Print and shaded views of the part. All mm, measured from the part's lowest x, y and z. A direction names the side the tool comes from. Round coordinates to 2 decimals unless told otherwise and drop trailing zeros. Write each loop counter-clockwise with the first axis right and the second up, starting at its lowest first coordinate (ties: lowest second). Pieces come first, ordered by that corner, then holes. Notation, with made-up numbers: M -35,81.5 L 7,81.5 A30 cw 7,114.5 Z; hole C -0.5,-26 d9. An arc over 180 degrees is marked long. Write item = value, one per line. Start each with the question number.
Q1. Probe L1, parallel to X at y = 15.25, z = 30.5; L2, parallel to Z at x = 44.5, y = 18.75; L3, parallel to Z at x = 54, y = 18.25. List the from-to ranges inside material, lowest first.
Q2. Band-saw the part on B-B on z = 36.5. Write the cut outline in (x, y), plus the area to 3 significant figures.
Q3. Pull direction Z, two halves, no side cores. Call the marked faces 1, 2, 3 and 4: released by +Z, released by -Z, zero draft, split by the parting line, or undercut.
Q4. Band-saw the part on C-C on y = 8.75. Write the cut outline in (x, z).
Q5. Band-saw the part on D-D on z = 10. Write the cut outline in (x, y), plus the area to 3 significant figures.
Q6. Drop flat-ended pins along their axis: P1, Ø2, axis at x = 13, y = 5, coming from the +Z side; P2, Ø4, axis at x = 38.5, y = 22.5, coming from the -Z side; P3, Ø6.5, axis at y = 13.5, z = 21, coming from the +X side. Give the stop position or say it passes through.
Q7. Tool access for the marked faces 5, 6, 7 and 8: list every direction of +Z, -Z, +X, -X, +Y, -Y with a clear straight run to the whole face (end or side of a thin tool).
Q8. Band-saw the part on A-A on x = 57.5. Write the cut outline in (y, z).
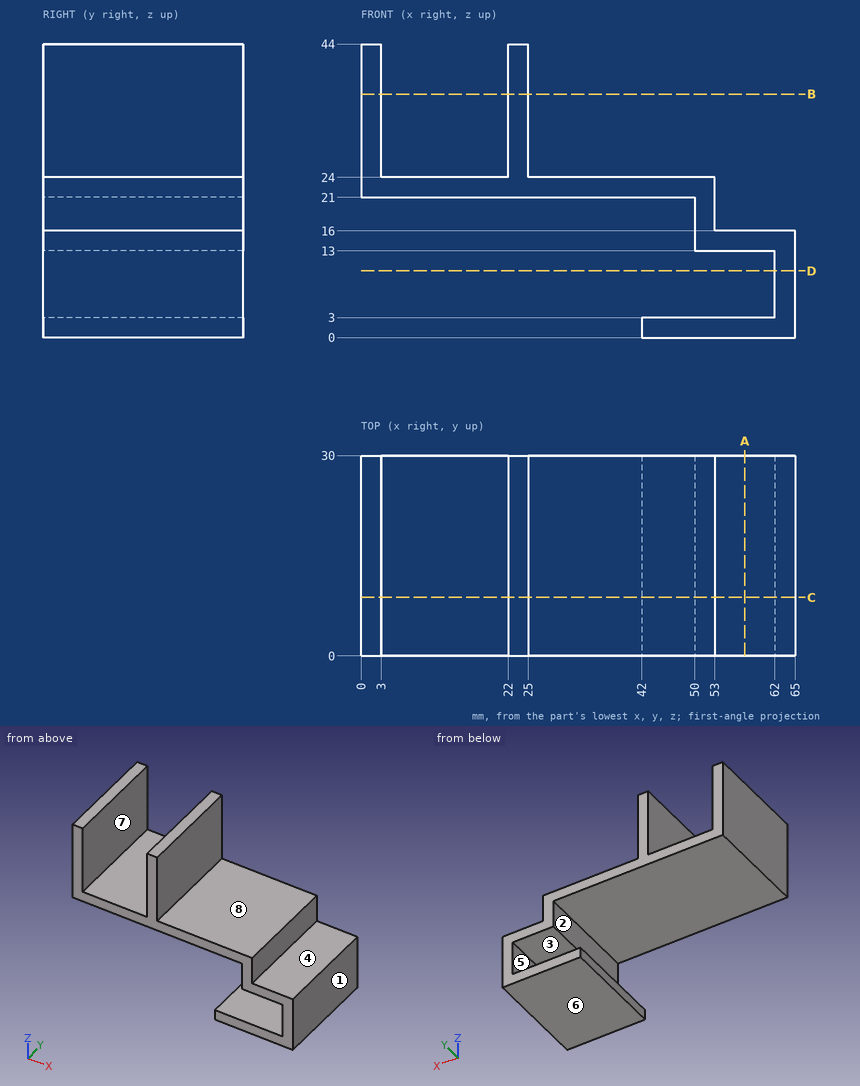
Conclusion:
q1.L1 = 0 to 3, 22 to 25
q1.L2 = 0 to 3, 21 to 24
q1.L3 = 0 to 3, 13 to 16
q2.outline = M 0,0 L 3,0 L 3,30 L 0,30 Z; M 22,0 L 25,0 L 25,30 L 22,30 Z
q2.area = 180 mm^2
q3.face_1 = zero draft
q3.face_2 = undercut
q3.face_3 = undercut
q3.face_4 = released by +Z
q4.outline = M 0,21 L 50,21 L 50,13 L 62,13 L 62,3 L 42,3 L 42,0 L 65,0 L 65,16 L 53,16 L 53,24 L 25,24 L 25,44 L 22,44 L 22,24 L 3,24 L 3,44 L 0,44 Z
q5.outline = M 62,0 L 65,0 L 65,30 L 62,30 Z
q5.area = 90.0 mm^2
q6.P1 = 24
q6.P2 = 21
q6.P3 = 53
q7.face_5 = -X, +Y, -Y
q7.face_6 = -Z, +X, -X, +Y, -Y
q7.face_7 = +Z, +Y, -Y
q7.face_8 = +Z, +X, +Y, -Y
q8.outline = M 0,0 L 30,0 L 30,3 L 0,3 Z; M 0,13 L 30,13 L 30,16 L 0,16 Z
